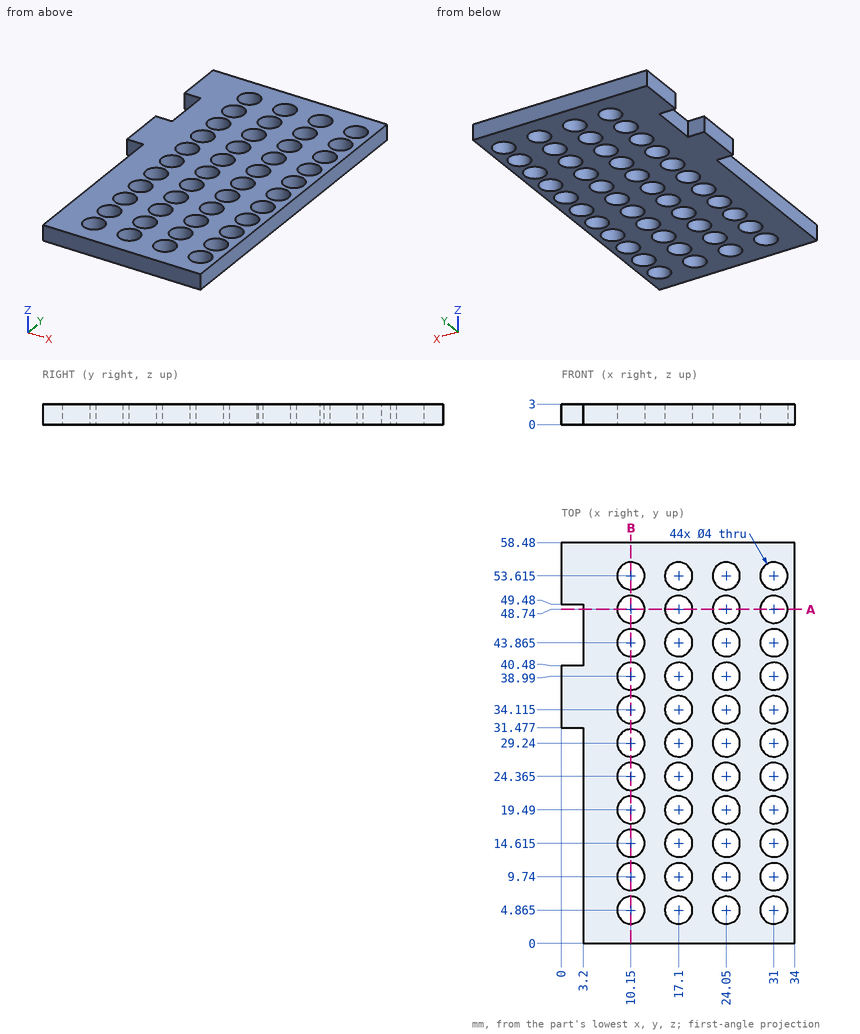
Can you work these out from the drawing? Everything is in mm from the part's minimum corner. Coordinates: 2 decimals unless noted, no trailing zeros. Loops run counter-clockwise (first coordinate to the right, second up) from the corner with the lowest first, then second, coordinate; pieces in that order, holes last.
1) For pin 1 (3 mm diameter, centred on x = 10.15, y = 4.865, fed in from +Z), with a flat end and sliding along its axis, tell me the tip position at first contact or that it passes through.
2) I need wall thicknesses on probe 1 along X at (y, z) = (29, 0.4) (1 decimal); probe 2 along X at (y, z) = (27.5, 2.05) (1 decimal); probe 3 along Y at (x, z) = (20, 2.4). Which ranges of each line are inside material? Lowest first, please.
3) Imagine slicing it at B-B on x = 10.15. State how many separate pieces and enclosed holes the cut face has.
4) Imagine slicing it at A-A on y = 48.74. List the corners of the cut face in (x, z) for me.
Completed:
1. pin 1: passes through
2. probe 1: x = 3.2 to 8.2, 12.1 to 15.1, 19.1 to 22.1, 26 to 29, 33 to 34
2. probe 2: x = 3.2 to 9.2, 11.1 to 16.1, 18.1 to 23.1, 25 to 30, 32 to 34
2. probe 3: y = 0 to 58.48
3. separate pieces: 12
3. enclosed holes: 0
4. outline: (3.2, 0) - (8.15, 0) - (8.15, 3) - (3.2, 3) - close; (12.15, 0) - (15.1, 0) - (15.1, 3) - (12.15, 3) - close; (19.1, 0) - (22.05, 0) - (22.05, 3) - (19.1, 3) - close; (26.05, 0) - (29, 0) - (29, 3) - (26.05, 3) - close; (33, 0) - (34, 0) - (34, 3) - (33, 3) - close
